Part model, mm, in its own coordinate system. A direction names the side the tool comes from. Give positions to 0.01 mm unless a question says otherwise; leave off trailing zeros. Write each loop counter-clockwise with the first axis right and the second up, starting at its lowest first coordinate (ties: lowest second). Pieces come first, ordered by that corner, then holes. Notation, with made-up numbers: M 9.5,16.25 L 36.5,16.25 A10 ccw 36.5,25.25 Z; hole C 82.5,-11.75 d9. An arc over 180 degrees is marked long. Use a Markdown table: item, result.
```python
from build123d import *

# Parameters (mm, degrees)
F0_R     = 1.569142
F0_R_2   = 1.625806
F1_DEPTH = 0.508


with BuildPart() as f1:
    # F0 (on Top) → F1 (new body)
    with BuildSketch(Plane.XY):
        with BuildLine():
            Line((-6.436094, 45.351289), (-9.320162, 45.351289))
            ThreePointArc((-9.320162, 45.351289), (-11.235743, 45.055465), (-12.972845, 44.195556))
            ThreePointArc((-12.972845, 44.195556), (-14.955631, 41.927717), (-15.670162, 39.001289))
            Line((-15.670162, 39.001289), (-15.670162, -38.632582))
            ThreePointArc((-15.670162, -38.632582), (-13.81029, -43.12271), (-9.320162, -44.982582))
            Line((-9.320162, -44.982582), (6.739195, -44.982582))
            ThreePointArc((6.739195, -44.982582), (11.229323, -43.12271), (13.089195, -38.632582))
            Line((13.089195, -38.632582), (13.089195, 39.001289))
            ThreePointArc((13.089195, 39.001289), (12.505726, 41.660164), (10.862544, 43.830419))
            ThreePointArc((10.862544, 43.830419), (8.93664, 44.958951), (6.739195, 45.351289))
            Line((6.739195, 45.351289), (4.366797, 45.351289))
            Line((4.366797, 45.351289), (-6.436094, 45.351289))
        make_face()
        with BuildLine():
            Line((0.10242, -37.239678), (-1.945966, -37.239678))
            ThreePointArc((-1.945966, -37.239678), (-6.436094, -35.379806), (-8.295966, -30.889678))
            Line((-8.295966, -30.889678), (-8.295966, 30.152257))
            ThreePointArc((-8.295966, 30.152257), (-7.812601, 32.582297), (-6.436094, 34.642385))
            Line((-6.436094, 34.642385), (-6.436094, 26.376916))
            Line((-6.436094, 26.376916), (-6.436094, -28.02352))
            Line((-6.436094, -28.02352), (4.366797, -28.02352))
            Line((4.366797, -28.02352), (4.366797, 26.376916))
            Line((4.366797, 26.376916), (4.366797, 34.642385))
            Line((4.366797, 34.642385), (4.366797, 34.857317))
            ThreePointArc((4.366797, 34.857317), (4.441516, 34.7885), (4.515124, 34.718497))
            ThreePointArc((4.515124, 34.718497), (5.948067, 32.632361), (6.45242, 30.152257))
            Line((6.45242, 30.152257), (6.45242, -30.889678))
            ThreePointArc((6.45242, -30.889678), (4.592548, -35.379806), (0.10242, -37.239678))
        make_face(mode=Mode.SUBTRACT)
        with BuildLine():
            ThreePointArc((-12.972845, 44.195556), (-11.235743, 45.055465), (-9.320162, 45.351289))
            Line((-9.320162, 45.351289), (-6.436094, 45.351289))
            Line((-6.436094, 45.351289), (4.366797, 45.351289))
            Line((4.366797, 45.351289), (6.739195, 45.351289))
            ThreePointArc((6.739195, 45.351289), (8.93664, 44.958951), (10.862544, 43.830419))
            ThreePointArc((10.862544, 43.830419), (-0.850933, 57.343891), (-12.972845, 44.195556))
        make_face()
        with Locations((-4.932173, 52.845966)):
            Circle(F0_R, mode=Mode.SUBTRACT)
        with BuildLine():
            ThreePointArc((1.846396, 49.016528), (-1.102735, 45.801074), (-4.051865, 49.016528))
            Line((-4.051865, 49.016528), (1.846396, 49.016528))
        make_face(mode=Mode.SUBTRACT)
        with Locations((3.237295, 53.016163)):
            Circle(F0_R_2, mode=Mode.SUBTRACT)
    extrude(amount=F1_DEPTH)


solid = f1.part
```
1. Tool access for faces 5 (the cylindrical face through (-6.386, -35.429, 0.25)), 6 (the flat face through (-1, 7, 0)): list every direction of +Z, -Z, +X, -X, +Y, -Y with a clear straight run to the whole face (end or side of a thin tool).
Findings below:
| item | result |
|---|---|
| face 5 | +Z, -Z |
| face 6 | -Z, +X, -X, +Y, -Y |
2. Cut at C-C, the plane z = 0.15. Give the cut face in (x, y).
Findings below:
| item | result |
|---|---|
| outline | M -15.67,-38.63 A6.35 ccw -9.32,-44.98 L 6.74,-44.98 A6.35 ccw 13.09,-38.63 L 13.09,39 A6.35 ccw 10.86,43.83 A11.99 ccw long -12.97,44.2 A6.35 ccw -15.67,39 Z; hole M -8.3,-30.89 A6.35 ccw -1.95,-37.24 L 0.1,-37.24 A6.35 ccw 6.45,-30.89 L 6.45,30.15 A6.35 ccw 4.52,34.72 A6.35 ccw 4.37,34.86 L 4.37,-28.02 L -6.44,-28.02 L -6.44,34.64 A6.35 ccw -8.3,30.15 Z; hole C -4.93,52.85 d3.14; hole M -4.05,49.02 A2.96 ccw long 1.85,49.02 Z; hole C 3.24,53.02 d3.25 |
3. Cut at A-A, the plane y = -27. Give the cut face in (x, z).
Findings below:
| item | result |
|---|---|
| outline | M -15.67,0 L -8.3,0 L -8.3,0.51 L -15.67,0.51 Z; M -6.44,0 L 4.37,0 L 4.37,0.51 L -6.44,0.51 Z; M 6.45,0 L 13.09,0 L 13.09,0.51 L 6.45,0.51 Z |
4. Two-plate mould, pull along X, no slides. Class faces 1 (the cylindrical face through (-7.826, 32.55, 0.25)), 2 (the cylindrical face through (12.52, 41.63, 0.25)), 3 (the cylindrical face through (-13.86, -43.07, 0.25)), 4 (the cylindrical face through (4.64, -35.33, 0.25)): released by +X, released by -X, zero draft, split by the parting line, or undercut.
Findings below:
| item | result |
|---|---|
| face 1 | undercut |
| face 2 | released by +X |
| face 3 | released by -X |
| face 4 | undercut |
5. Cut at B-B, the plane x = 3. Give the cut face in (y, z).
Findings below:
| item | result |
|---|---|
| outline | M -44.98,0 L -36.54,0 L -36.54,0.51 L -44.98,0.51 Z; M -28.02,0 L 51.41,0 L 51.41,0.51 L -28.02,0.51 Z; M 54.62,0 L 56.65,0 L 56.65,0.51 L 54.62,0.51 Z |
6. Drill centre lines: L1, parallel to X at y = 27.5, z = 0.4; L2, parallel to Y at x = 3.5, z = 0.45; L3, parallel to X at y = -28.5, z = 0.1. Where is each one in solid material? Low to high.
Findings below:
| item | result |
|---|---|
| L1 | -15.67 to -8.3, -6.44 to 4.37, 6.45 to 13.09 |
| L2 | -44.98 to -36.25, -28.02 to 51.41, 54.62 to 56.46 |
| L3 | -15.67 to -8.3, 6.45 to 13.09 |
